from build123d import *

# Parameters (mm, degrees)
CROQUIS1_R              = 7
SALIENTE_EXTRUIR1_DEPTH = 5
CROQUIS2_R              = 2.5
CORTAR_EXTRUIR1_DEPTH   = 5
CROQUIS3_R              = 6
CROQUIS3_R_2            = 4
CORTAR_EXTRUIR3_DEPTH   = 0.5
CROQUIS4_R              = 6
CROQUIS4_R_2            = 4
CORTAR_EXTRUIR4_DEPTH   = 0.5
CHAFL_N1_SIZE           = 0.2


with BuildPart() as part:
    # Croquis1 → Saliente-Extruir1 (new body)
    with BuildSketch(Plane.XY):
        Circle(CROQUIS1_R)
    extrude(amount=SALIENTE_EXTRUIR1_DEPTH)

    # Croquis2 → Cortar-Extruir1 (cut)
    with BuildSketch(Plane.XY.offset(5)):
        Circle(CROQUIS2_R)
    extrude(amount=-CORTAR_EXTRUIR1_DEPTH, mode=Mode.SUBTRACT)

    # Croquis3 → Cortar-Extruir3 (cut)
    with BuildSketch(Plane.XY.offset(5)):
        Circle(CROQUIS3_R)
        Circle(CROQUIS3_R_2, mode=Mode.SUBTRACT)
    extrude(amount=-CORTAR_EXTRUIR3_DEPTH, mode=Mode.SUBTRACT)

    # Croquis4 → Cortar-Extruir4 (cut)
    with BuildSketch(Plane(origin=(0, 0, 0), x_dir=(-1, 0, 0), z_dir=(0, 0, -1))):
        Circle(CROQUIS4_R)
        Circle(CROQUIS4_R_2, mode=Mode.SUBTRACT)
    extrude(amount=-CORTAR_EXTRUIR4_DEPTH, mode=Mode.SUBTRACT)

    # Chaflán1
    chafl_n1_edges = [part.edges().sort_by_distance(p)[0] for p in [
        (-6, 0, 5),
        (-4, 0, 5),
        (-7, 0, 0),
        (6, 0, 0),
        (4, 0, 0),
        (-7, 0, 5),
        (-2.5, 0, 0),
        (-2.5, 0, 5),
    ]]
    chamfer(chafl_n1_edges, length=CHAFL_N1_SIZE)


solid = part.part
Here's how the part is built. I have some questions about the finished solid (model axes, mm). A direction names the side the tool comes from. Give positions to 0.01 mm unless a question says otherwise; leave off trailing zeros. Loops run counter-clockwise (first coordinate to the right, second up) from the corner with the lowest first, then second, coordinate; pieces in that order, holes last. Notation, with made-up numbers: (-16, -31.75) -> (29, -31.75) arc R14 ccw to (29, -18.75) -> close; hole circle Ø11 at (-10, -40). An arc over 180 degrees is marked (long way). One line per item, written item: value.
Q1. If I drill on line 1 along Y through (x, z) = (0, 0.3); line 2 along Y through (x, z) = (3.25, 3.8); line 3 along Z through (x, y) = (4.5, 1.5), over which ranges is the centre line in solid material (lowest first)?
Answers follow:
line 1: -7 to -6, -4 to -2.5, 2.5 to 4, 6 to 7
line 2: -6.2 to 6.2
line 3: 0.5 to 4.5
Q2. I'm going to push flat-ended pins straight in: pin 1 Ø2 at (x, y) = (4, -4.5) entering from -Z; pin 2 Ø1 at (y, z) = (2, 3.5) entering from -X. Where does each tip first touch, or does it pass through?
Answers follow:
pin 1: z = 0
pin 2: x = -6.84
Q3. We'd pull the mould along X, two halves only. Please class faces 1 (the face through (6.466, -2.681, 2.468)), 2 (the face through (1, 3, 0)), 3 (the face through (-0.54, -2.44, 2.53)): pulls with the +X half, pulls with the -X half, needs draft (parallel to the pull), parting line crosses it, or undercut.
Answers follow:
face 1: parting line crosses it
face 2: needs draft
face 3: undercut
Q4. On a 3-axis mill with a long thin cutter (end or side, diameter ignored), from which of +Z, -Z, +X, -X, +Y, -Y can I reach the whole of each face in a straight line? I mean faces 4 (the face through (1.42, -3.92, 0.5)), 5 (the face through (-4.76, -3.65, 4.65)), 6 (the face through (1, 3, 5)). Say none if no direction works.
Answers follow:
face 4: -Z
face 5: +Z
face 6: +Z, +X, -X, +Y, -Y
Q5. Suppose I cut it at A-A on z = 1.65. Please give me the cut outline in (x, y).
Answers follow:
outline: circle Ø14 at (0, 0); hole circle Ø5 at (0, 0)
